Can you work these out from the drawing? Everything is in mm from the part's minimum corner. A direction names the side the tool comes from. Round coordinates to 2 decimals unless told otherwise and drop trailing zeros. Order: outer loops, then holes, each group sorted by start corner. A loop starts at its lowest first (then second) coordinate and runs counter-clockwise, first axis right, second up. Notation, with made-up numbers: (-39, -22.5) -> (-28, -22.5) arc R36 cw to (-28, 13.5) -> close; hole circle Ø3 at (44.25, 36). An arc over 180 degrees is marked (long way). One line per item, written item: value.
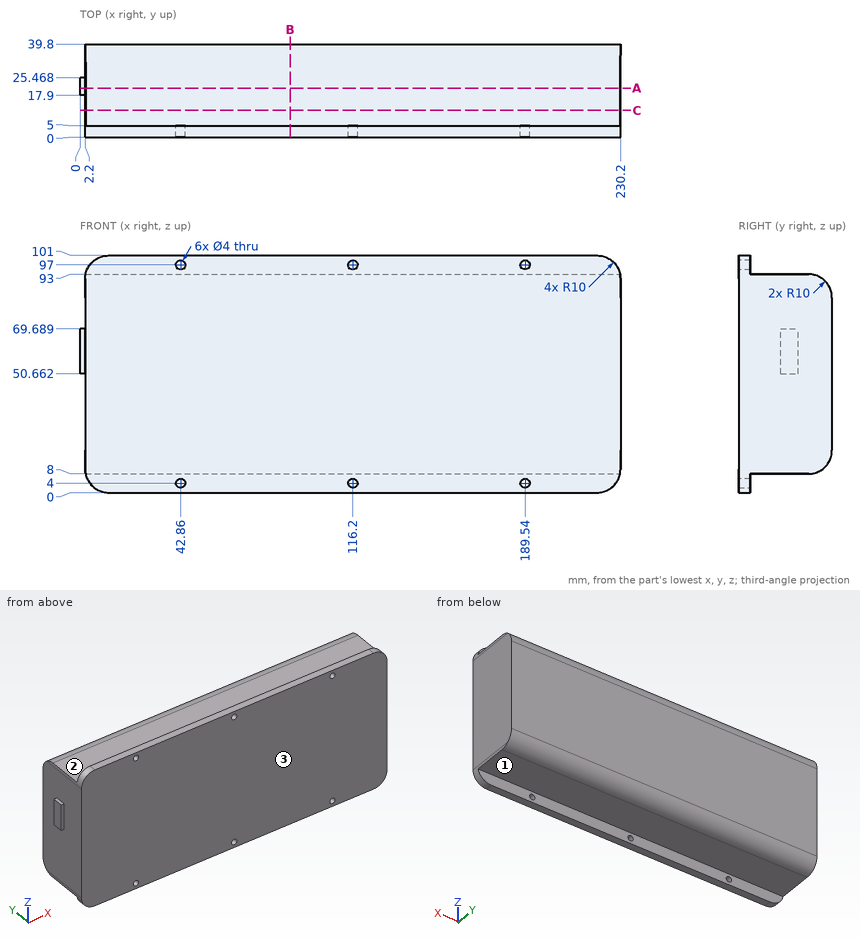
Q1. For P1, Ø2.5, axis at x = 0.5, z = 56, coming from the -Y side; P2, Ø9, axis at x = 103.5, z = 98, coming from the +Y side; P3, Ø1.1, axis at x = 1, z = 59.5, coming from the +Y side, each with a flat end and sliding along its axis, tell me the tip position at first contact or that it passes through.
Answers:
P1: y = 17.9
P2: y = 5
P3: y = 25.47
Q2. I want a section at C-C on y = 11.5. Write out the boundary of the cut face in (x, z).
Answers:
outline: (2.2, 10) arc R10 ccw to (2.4, 8) -> (230, 8) arc R10 ccw to (230.2, 10) -> (230.2, 91) arc R10 ccw to (230, 93) -> (2.4, 93) arc R10 ccw to (2.2, 91) -> close
Q3. I want a section at A-A on y = 21. Write out the boundary of the cut face in (x, z).
Answers:
outline: (0, 50.66) -> (2.2, 50.66) -> (2.2, 10) arc R10 ccw to (2.4, 8) -> (230, 8) arc R10 ccw to (230.2, 10) -> (230.2, 91) arc R10 ccw to (230, 93) -> (2.4, 93) arc R10 ccw to (2.2, 91) -> (2.2, 69.69) -> (0, 69.69) -> close
Q4. I want a section at B-B on x = 89.5. Write out the boundary of the cut face in (y, z), then the cut area to 3 significant figures.
Answers:
outline: (0, 0) -> (5, 0) -> (5, 8) -> (29.8, 8) arc R10 ccw to (39.8, 18) -> (39.8, 83) arc R10 ccw to (29.8, 93) -> (5, 93) -> (5, 101) -> (0, 101) -> close
area: 3,420 mm2
Q5. I need wall thicknesses on line 1 along Z through (x, y) = (116.2, 3.1); line 2 along X through (y, z) = (2, 97); line 3 along Z through (x, y) = (42, 2) (1 decimal). Which ranges of each line are inside material? Lowest first, please.
Answers:
line 1: 0 to 2, 6 to 95, 99 to 101
line 2: 4.2 to 40.86, 44.86 to 114.2, 118.2 to 187.54, 191.54 to 228.2
line 3: 0 to 2.2, 5.8 to 95.2, 98.8 to 101
Q6. Which directions (+Z, -Z, +X, -X, +Y, -Y) give clear straight access to the entire face, cutting with the end or side of a thin tool? Please do the marked faces 1, 2 and 3.
Answers:
face 1: -Z, +X, -X, +Y
face 2: +Z, +X, -X, +Y
face 3: +Z, -Z, +X, -X, -Y
